For this review, use the dimensioned drawing (mm, ordinates from the lowest corner) and the shaded views. A direction names the side the tool comes from. Coordinates: 2 decimals unless noted, no trailing zeros. Order: outer loops, then holes, each group sorted by start corner. A loop starts at its lowest first (then second) coordinate and runs counter-clockwise, first axis right, second up. Notation, with made-up numbers: M 64.5,64 L 79.5,64 A21 cw 79.5,75 Z; hole C 25.5,63 d7. An arc over 180 degrees is marked long. Answer as CSV lines item,"result". Start each with the question number.
Q1. Consider section C-C on z = 4.5. Write out the cut boundary in (x, y), and give its area (3 significant figures).
Q2. For P1, Ø3, axis at x = 7, z = 9.5, coming from the +Y side; P2, Ø2.5, axis at x = 29.6, z = 5.9, coming from the +Y side; P3, Ø3.5, axis at x = 22.5, z = 8.5, coming from the +Y side; P4, Ø2, axis at x = 12, z = 5.5, coming from the -Y side, all flat-tipped, find the tip position at first contact; note any pin that passes through.
Q3. Consider section B-B on x = 12.5. Write out the cut boundary in (y, z).
Q4. Consider section A-A on x = 29.6. Write out the cut boundary in (y, z), and give its area (3 significant figures).
Q5. Consider section D-D on y = 27.5. Write out the cut boundary in (x, z).
Q6. Machinability: for the marked faces 1, 2 and 3, which of the approach directions +Z, -Z, +X, -X, +Y, -Y give a long, thin tool a straight path to every point of the face, cutting with its end or side? Answer none if there is none.
Q7. Wall thickness on L1, parallel to X at y = 17.3, z = 5.9; L2, parallel to Z at x = 2.3, y = 16.65; L3, parallel to X at y = 4, z = 1: over which ranges is each line inside the solid? List them lowest first. Write a range as [from, to].
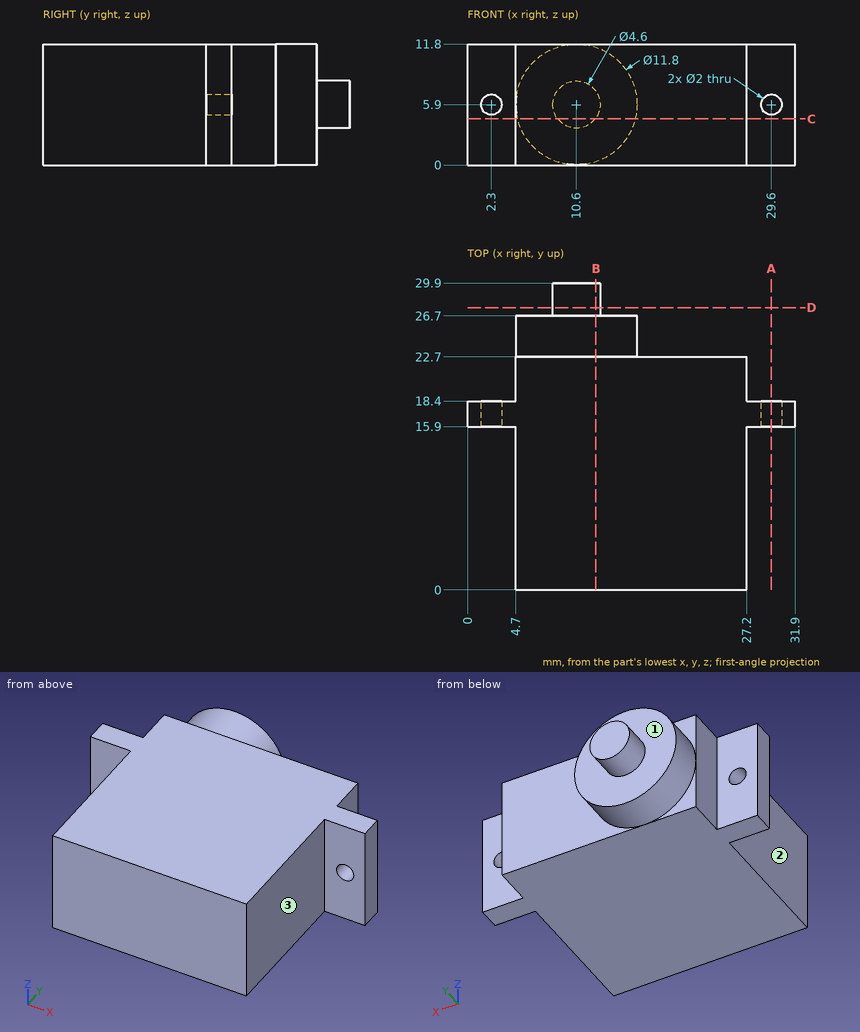
Evaluation:
1,outline,"M 0,15.9 L 4.7,15.9 L 4.7,0 L 27.2,0 L 27.2,15.9 L 31.9,15.9 L 31.9,18.4 L 27.2,18.4 L 27.2,22.7 L 16.33,22.7 L 16.33,26.7 L 12.42,26.7 L 12.42,29.9 L 8.78,29.9 L 8.78,26.7 L 4.87,26.7 L 4.87,22.7 L 4.7,22.7 L 4.7,18.4 L 0,18.4 Z"
1,area,"592 mm²"
2,P1,"stops at y = 26.7"
2,P2,"stops at y = 18.4"
2,P3,"stops at y = 22.7"
2,P4,"stops at y = 0"
3,outline,"M 0,0 L 22.7,0 L 22.7,0.31 L 26.7,0.31 L 26.7,4.6 L 29.9,4.6 L 29.9,7.2 L 26.7,7.2 L 26.7,11.49 L 22.7,11.49 L 22.7,11.8 L 0,11.8 Z"
4,outline,"M 15.9,0 L 18.4,0 L 18.4,4.9 L 15.9,4.9 Z; M 15.9,6.9 L 18.4,6.9 L 18.4,11.8 L 15.9,11.8 Z"
4,area,"24.5 mm²"
5,outline,"C 10.6,5.9 d4.6"
6,face 1,"+Y"
6,face 2,"+Z, -Z, -X, -Y"
6,face 3,"+Z, -Z, +X, -Y"
7,L1,"x = [0, 1.3], [3.3, 28.6], [30.6, 31.9]"
7,L2,"z = [0, 4.9], [6.9, 11.8]"
7,L3,"x = [4.7, 27.2]"
